Can you work these out from the model? Positions are in its coordinate system, mm. A direction names the side the tool comes from. Coordinates: 2 decimals unless noted, no trailing zeros. Write each loop counter-clockwise with the first axis right and the second up, starting at its lowest first coordinate (ties: lowest second). Pieces come first, ordered by that corner, then holes. Notation, with made-up numbers: (78.25, 30.5) -> (101.25, 30.5) arc R13 cw to (101.25, 53.5) -> close; hole circle Ø5 at (45, -10.5). An arc over 180 degrees is marked (long way). Use one line per item in the form item = value.
```python
from build123d import *

# Parameters (mm, degrees)
SKETCH3_W           = 63.5
SKETCH3_H           = 76.2
BOSS_EXTRUDE2_DEPTH = 2.54
SKETCH4_R           = 17.270000004
SKETCH4_R_2         = 16.000000004
BOSS_EXTRUDE3_DEPTH = 10
SKETCH5_R           = 13.983999972
CUT_EXTRUDE1_DEPTH  = 10.0076
SKETCH8_R           = 2.032
CUT_EXTRUDE2_DEPTH  = 3.54
SKETCH9_W           = 10.16
SKETCH9_H           = 3.81
BOSS_EXTRUDE4_DEPTH = 1.016


with BuildPart() as part:
    # Sketch3 → Boss-Extrude2 (new body)
    with BuildSketch(Plane.XY):
        with Locations((31.75, 38.1)):
            Rectangle(SKETCH3_W, SKETCH3_H)
    extrude(amount=BOSS_EXTRUDE2_DEPTH)

    # Sketch4 → Boss-Extrude3 (add)
    with BuildSketch(Plane(origin=(0, 0, 0), x_dir=(-1, 0, 0), z_dir=(0, 0, -1))):
        with Locations((-31.75, 38.1)):
            Circle(SKETCH4_R)
        with Locations((-31.75, 38.1)):
            Circle(SKETCH4_R_2, mode=Mode.SUBTRACT)
    extrude(amount=BOSS_EXTRUDE3_DEPTH)

    # Sketch5 → Cut-Extrude1 (cut)
    with BuildSketch(Plane(origin=(0, 0, 0), x_dir=(-1, 0, 0), z_dir=(0, 0, -1))):
        with Locations((-31.75, 38.1)):
            Circle(SKETCH5_R)
    extrude(amount=-CUT_EXTRUDE1_DEPTH, mode=Mode.SUBTRACT)

    # Sketch8 → Cut-Extrude2 (cut, through all)
    with BuildSketch(Plane(origin=(0, 0, 0), x_dir=(-1, 0, 0), z_dir=(0, 0, -1))):
        with Locations((-3.375, 63.5)):
            Circle(SKETCH8_R)
        with Locations((-60.125, 63.5)):
            Circle(SKETCH8_R)
        with Locations((-60.125, 12.7)):
            Circle(SKETCH8_R)
        with Locations((-3.375, 12.7)):
            Circle(SKETCH8_R)
    extrude(amount=-CUT_EXTRUDE2_DEPTH, mode=Mode.SUBTRACT)

    # Sketch9 → Boss-Extrude4 (add)
    with BuildSketch(Plane.XY.offset(2.54)):
        with Locations((51.6636, 50.165)):
            Rectangle(SKETCH9_W, SKETCH9_H)
        with Locations((11.8364, 50.165)):
            Rectangle(SKETCH9_W, SKETCH9_H)
    extrude(amount=BOSS_EXTRUDE4_DEPTH)


solid = part.part
```
Q1. Will these pins go through, and if not, where does the flat tip stop? pin 1 (3 mm diameter, centred on x = 13.5, y = 59, fed in from +Z); pin 2 (1.1 mm diameter, centred on x = 12, z = 3.5, fed in from +Y); pin 3 (0.8 mm diameter, centred on y = 49.5, z = 3.5, fed in from +X); pin 4 (17 mm diameter, centred on x = 31.75, y = 38.1, fed in from +Z).
Return value:
pin_1 = 2.54
pin_2 = 52.07
pin_3 = 56.74
pin_4 = through
Q2. Thinking about a two-plate mould opening in X: for faces 3 (the flat face through (31, 76.2, 1)), 4 (the cylindrical face through (62.155, 12.789, 1.252)), 5 (the flat face through (31.68, 23.95, 0)), 6 (the flat face through (63.5, 38, 1)), which applies, released by +X, released by -X, zero draft, split by the parting line, or undercut?
Return value:
face_3 = zero draft
face_4 = undercut
face_5 = undercut
face_6 = released by +X
Q3. If I drill on line 1 (X direction, y = 11, z = 2); line 2 (Y direction, x = 31.75, z = -2.25); line 3 (Z direction, x = 4, y = 71.5), over which ranges is the centre line in solid material (lowest first)? Write a range as from..to.
Return value:
line_1 = 0..2.26, 4.49..59.01, 61.24..63.5
line_2 = 20.83..22.1, 54.1..55.37
line_3 = 0..2.54
Q4. Suppose I cut it at D-D (z = -1.5). Write out the boundary of the cut face in (x, y), then the cut area to 3 significant figures.
Return value:
outline = circle Ø34.54 at (31.75, 38.1); hole circle Ø32 at (31.75, 38.1)
area = 133 mm2
Q5. Suppose I cut it at B-B (x = 31.75). Write out the boundary of the cut face in (y, z).
Return value:
outline = (0, 0) -> (20.83, 0) -> (20.83, -10) -> (22.1, -10) -> (22.1, 0) -> (24.12, 0) -> (24.12, 2.54) -> (0, 2.54) -> close; (52.08, 0) -> (54.1, 0) -> (54.1, -10) -> (55.37, -10) -> (55.37, 0) -> (76.2, 0) -> (76.2, 2.54) -> (52.08, 2.54) -> close
Q6. Suppose I cut it at C-C (y = 12.7). Write out the boundary of the cut face in (x, z).
Return value:
outline = (0, 0) -> (1.34, 0) -> (1.34, 2.54) -> (0, 2.54) -> close; (5.41, 0) -> (58.09, 0) -> (58.09, 2.54) -> (5.41, 2.54) -> close; (62.16, 0) -> (63.5, 0) -> (63.5, 2.54) -> (62.16, 2.54) -> close
Q7. Suppose I cut it at A-A (y = 38.1). Write out the boundary of the cut face in (x, z).
Return value:
outline = (0, 0) -> (14.48, 0) -> (14.48, -10) -> (15.75, -10) -> (15.75, 0) -> (17.77, 0) -> (17.77, 2.54) -> (0, 2.54) -> close; (45.73, 0) -> (47.75, 0) -> (47.75, -10) -> (49.02, -10) -> (49.02, 0) -> (63.5, 0) -> (63.5, 2.54) -> (45.73, 2.54) -> close
Q8. For faces 1 (the cylindrical face through (3.64, 65.515, 1.252)), 2 (the cylindrical face through (45.455, 27.591, -4.93)), which set-ups out of +Z, -Z, +X, -X, +Y, -Y let a thin tool reach every point of the face, with its end or its side?
Return value:
face_1 = +Z, -Z
face_2 = -Z
